from build123d import *

# Parameters (mm, degrees)
F1_R     = 2
F3_DEPTH = 8.4
F5_R     = 2
F6_DEPTH = 25
F7_DEPTH = 1.7
F8_R     = 1


with BuildPart() as f3:
    # F1 (on Top) → F3 (new body, through all)
    with BuildSketch(Plane.XY):
        with BuildLine():
            Line((9.5, 6.25), (1.7853571071, 6.25))
            ThreePointArc((1.7853571071, 6.25), (5.1891628032, 3.9144079248), (6.5, 0))
            ThreePointArc((6.5, 0), (5.1891628032, -3.9144079248), (1.7853571071, -6.25))
            Line((1.7853571071, -6.25), (9.5, -6.25))
            Line((9.5, -6.25), (9.5, 6.25))
        make_face()
        with BuildLine():
            Line((1.7853571071, 6.25), (-1.7853571071, 6.25))
            ThreePointArc((-1.7853571071, 6.25), (-6.5, 0), (-1.7853571071, -6.25))
            Line((-1.7853571071, -6.25), (1.7853571071, -6.25))
            ThreePointArc((1.7853571071, -6.25), (5.1891628032, -3.9144079248), (6.5, 0))
            ThreePointArc((6.5, 0), (5.1891628032, 3.9144079248), (1.7853571071, 6.25))
        make_face()
        Polygon((-3.7527767497, 0), (-1.8763883749, 3.25), (1.8763883749, 3.25), (3.7527767497, 0), (1.8763883749, -3.25), (-1.8763883749, -3.25), align=None, mode=Mode.SUBTRACT)
        Polygon((1.8763883749, 3.25), (-1.8763883749, 3.25), (-3.7527767497, 0), (-1.8763883749, -3.25), (1.8763883749, -3.25), (3.7527767497, 0), align=None)
        Circle(F1_R, mode=Mode.SUBTRACT)
    extrude(amount=F3_DEPTH)

    # F2 (on Front) → F4 (revolve, cut)
    with BuildSketch(Plane.XZ):
        Polygon((0, 6.2), (0, 1.7), (6.5, 1.7), (6.5, 6.7), (3.2177651569, 6.7), (2.7, 6.2), align=None)
    revolve(axis=Axis((0, 0, 4.2), (0, 0, 1)), mode=Mode.SUBTRACT)

    # F5 (on face) → F6 (cut)
    with BuildSketch(Plane.XY.offset(8.4)):
        Circle(F5_R)
    extrude(amount=-F6_DEPTH, mode=Mode.SUBTRACT)

    # F1 (on Top) → F7 (cut, through all)
    with BuildSketch(Plane.XY):
        Polygon((1.8763883749, 3.25), (-1.8763883749, 3.25), (-3.7527767497, 0), (-1.8763883749, -3.25), (1.8763883749, -3.25), (3.7527767497, 0), align=None)
        Circle(F1_R, mode=Mode.SUBTRACT)
    extrude(amount=F7_DEPTH, mode=Mode.SUBTRACT)

    # F8
    f8_edges = [f3.edges().sort_by_distance(p)[0] for p in [
        (1.785357, 6.25, 4.2),
        (1.785357, -6.25, 4.2),
    ]]
    fillet(f8_edges, radius=F8_R)


solid = f3.part
Input: part model. Units: mm. Frame: model coordinates. A direction names the side the tool comes from. Coordinates: 2 decimals unless noted, no trailing zeros. Write each loop counter-clockwise with the first axis right and the second up, starting at its lowest first coordinate (ties: lowest second). Pieces come first, ordered by that corner, then holes. Notation, with made-up numbers: M 37.25,-17.5 L 56.25,-17.5 A13 ccw 56.25,-12.5 Z; hole C 79,-11 d2. An arc over 180 degrees is marked long. Answer as a JSON object with one key per item and string values. Group by question number.
(1) Ray query, line 1 along Z through (x, y) = (6, 0.5); line 2 along X through (y, z) = (0, 7.25); line 3 along Y through (x, z) = (0, 7.4). Return the intervals inside material, ascending. Write a range as [from, to].
(2) Section C-C on z = 6.5. Output: boundary loops of the cut face in (x, y), plus the area to 3 significant figures.
(3) Section A-A on x = 0. Output: boundary loops of the cut face in (y, z), plus the area to 3 significant figures.
(4) Mould query, pull axis X, two halves, no side actions, for faces 1 (the face through (0, 3.25, 1)), 2 (the face through (3, 0, 8.4)), 3 (the face through (4.428, -5.622, 4.235)). Classes: pulls with the +X half, pulls with the -X half, needs draft (parallel to the pull), parting line crosses it, or undercut.
(5) Set-up query: faces 4 (the face through (2.83, 1.6, 0.84)), 5 (the face through (-2, -1, 6.2)), 6 (the face through (4.44, 5.65, 4.24)), 7 (the face through (-2, 3, 6.7)), 8 (the face through (6, 6.25, 4)). Return all of +Z, -Z, +X, -X, +Y, -Y with unobstructed straight access to the full face (end or side cutting, diameter ignored); none if empty.
(6) Section D-D on y = 5.75. Output: boundary loops of the cut face in (x, z).
(7) Section B-B on z = 1. Output: boundary loops of the cut face in (x, y), plus the area to 3 significant figures.
(8) Contact query for a flat-ended pin moving along its axis: P1, Ø2.5, axis at x = 0, y = -1, coming from the -Z side. Output: stop coordinate, or through.
Result set:
{
 "1": {"line 1": "z = [0, 1.7], [6.7, 8.4]", "line 2": "x = [-6.5, -2], [2, 9.5]", "line 3": "y = [-6.25, -2], [2, 6.25]"},
 "2": {"outline": "C 0,0 d6.02; M 4.64,-4.55 A1 ccw 5.36,-6.25 L 9.5,-6.25 L 9.5,6.25 L 5.36,6.25 A1 ccw 4.64,4.55 A6.5 cw Z; hole C 0,0 d4", "area": "65.4 mm2"},
 "3": {"outline": "M -6.25,0 L -3.25,0 L -3.25,1.7 L -6.25,1.7 Z; M -6.25,6.7 L -3.22,6.7 L -2.7,6.2 L -2,6.2 L -2,8.4 L -6.25,8.4 Z; M 2,6.2 L 2.7,6.2 L 3.22,6.7 L 6.25,6.7 L 6.25,8.4 L 2,8.4 Z; M 3.25,0 L 6.25,0 L 6.25,1.7 L 3.25,1.7 Z", "area": "25.6 mm2"},
 "4": {"face 1": "undercut", "face 2": "needs draft", "face 3": "pulls with the -X half"},
 "5": {"face 4": "-Z", "face 5": "-Z, -X, +Y, -Y", "face 6": "-X", "face 7": "none", "face 8": "+Z, -Z, +X, -X, +Y"},
 "6": {"outline": "M -3.03,0 L 9.5,0 L 9.5,8.4 L -3.03,8.4 L -3.03,6.7 L 4.49,6.7 L 4.49,1.7 L -3.03,1.7 Z"},
 "7": {"outline": "M -1.79,-6.25 L 9.5,-6.25 L 9.5,6.25 L -1.79,6.25 A6.5 ccw Z; hole M -3.75,0 L -1.88,-3.25 L 1.88,-3.25 L 3.75,0 L 1.88,3.25 L -1.88,3.25 Z", "area": "148 mm2"},
 "8": {"P1": "stops at z = 6.2"}
}
